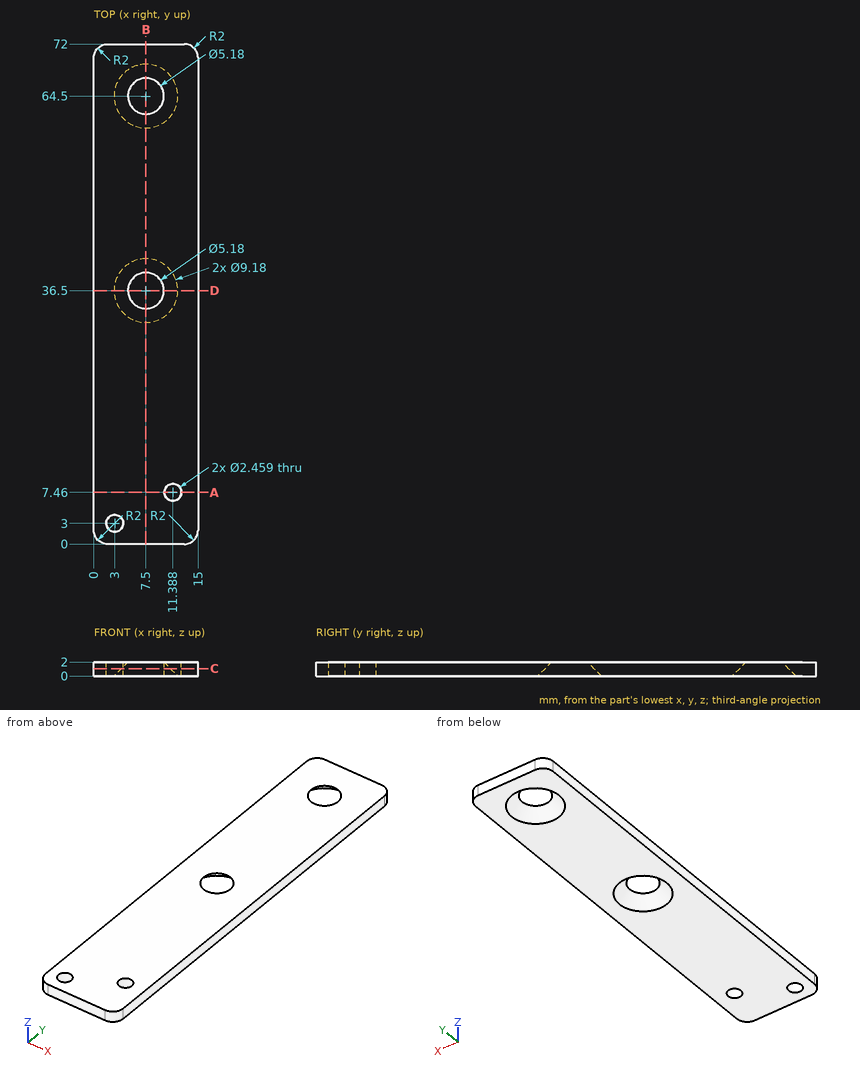
Here's the drawing with two shaded views (mm, measured from the low corner). I have some questions. Coordinates: 2 decimals unless noted, no trailing zeros. Order: outer loops, then holes, each group sorted by start corner. A loop starts at its lowest first (then second) coordinate and runs counter-clockwise, first axis right, second up. Notation, with made-up numbers: (-11.75, -24) - (47.25, -24) arc R13 ccw to (47.25, -4) - close; hole circle Ø11 at (-6.75, 61.25). An arc over 180 degrees is marked (long way). Use CSV: the item, a comma, the result in double quotes. Start each with the question number.
1. Suppose I cut it at B-B on x = 7.5. List the corners of the cut face in (y, z) for me, then the cut area to 3 significant figures.
2. Suppose I cut it at D-D on y = 36.5. List the corners of the cut face in (x, z) for me.
3. I'm going to push flat-ended pins straight in: pin 1 (4 mm diameter, centred on x = 10.5, y = 48.5, fed in from -Z); pin 2 (1.5 mm diameter, centred on x = 3, y = 3, fed in from +Z). Where does each tip first touch, or does it pass through?
4. Suppose I cut it at A-A on y = 7.46. List the corners of the cut face in (x, z) for me.
5. Suppose I cut it at C-C on z = 1.05. List the corners of the cut face in (x, y) for me.
6. Please list where these lines run through material, in increasing order: line 1 (X direction, y = 3, z = 1.55); line 2 (Y direction, x = 9.25, z = 0.5); line 3 (Y direction, x = 6, z = 1.2). Write a range as from..to.
Output:
1,outline,"(0, 0) - (31.91, 0) - (33.91, 2) - (0, 2) - close; (39.09, 2) - (41.09, 0) - (59.91, 0) - (61.91, 2) - close; (67.09, 2) - (69.09, 0) - (72, 0) - (72, 2) - close"
1,area,"115 mm2"
2,outline,"(0, 0) - (2.91, 0) - (4.91, 2) - (0, 2) - close; (10.09, 2) - (12.09, 0) - (15, 0) - (15, 2) - close"
3,pin 1,"stops at z = 0"
3,pin 2,"passes through"
4,outline,"(0, 0) - (10.16, 0) - (10.16, 2) - (0, 2) - close; (12.62, 0) - (15, 0) - (15, 2) - (12.62, 2) - close"
5,outline,"(0, 2) arc R2 ccw to (2, 0) - (13, 0) arc R2 ccw to (15, 2) - (15, 70) arc R2 ccw to (13, 72) - (2, 72) arc R2 ccw to (0, 70) - close; hole circle Ø2.46 at (3, 3); hole circle Ø7.08 at (7.5, 36.5); hole circle Ø7.08 at (7.5, 64.5); hole circle Ø2.46 at (11.39, 7.46)"
6,line 1,"x = 0..1.77, 4.23..15"
6,line 2,"y = 0..32.8, 40.2..60.8, 68.2..72"
6,line 3,"y = 0..33.46, 39.54..61.46, 67.54..72"
